from build123d import *

# Parameters (mm, degrees)
SKETCH1_R           = 1.4986
BOSS_EXTRUDE1_DEPTH = 6.731
BOSS_EXTRUDE2_DEPTH = 2.54
SKETCH3_W           = 2.54
SKETCH3_H           = 3.283466221
BOSS_EXTRUDE3_DEPTH = 8.0264


with BuildPart() as part:
    # Sketch1 → Boss-Extrude1 (new body)
    with BuildSketch(Plane.XY):
        Circle(SKETCH1_R)
    extrude(amount=BOSS_EXTRUDE1_DEPTH)

    # Sketch2 → Boss-Extrude2 (add)
    with BuildSketch(Plane(origin=(0, 0, 0), x_dir=(-1, 0, 0), z_dir=(0, 0, -1))):
        with BuildLine():
            Line((-1.74748007, -0.387866221), (-2.463536443, -0.387866221))
            ThreePointArc((-2.463536443, -0.387866221), (-2.643141566, -0.313471343), (-2.717536443, -0.133866221))
            Line((-2.717536443, -0.133866221), (-2.717536443, 3.1496))
            ThreePointArc((-2.717536443, 3.1496), (-2.345562055, 4.047625612), (-1.447536443, 4.4196))
            Line((-1.447536443, 4.4196), (1.417916008, 4.4196))
            ThreePointArc((1.417916008, 4.4196), (2.312179766, 4.051371774), (2.687871622, 3.160217845))
            Line((2.687871622, 3.160217845), (2.715395045, -0.131742652))
            ThreePointArc((2.715395045, -0.131742652), (2.641758277, -0.312718973), (2.461403923, -0.387866221))
            Line((2.461403923, -0.387866221), (1.74748007, -0.387866221))
            ThreePointArc((1.74748007, -0.387866221), (1.561141898, -0.306475854), (1.494222089, -0.114465319))
            ThreePointArc((1.494222089, -0.114465319), (0, 1.4986), (-1.494222089, -0.114465319))
            ThreePointArc((-1.494222089, -0.114465319), (-1.561141898, -0.306475854), (-1.74748007, -0.387866221))
        make_face()
    extrude(amount=-BOSS_EXTRUDE2_DEPTH)

    # Sketch3 → Boss-Extrude3 (add)
    with BuildSketch(Plane(origin=(2.717536443, 0, 0), x_dir=(0, 0, -1), z_dir=(1, 0, 0))):
        with Locations((-1.27, 1.50786689)):
            Rectangle(SKETCH3_W, SKETCH3_H)
    extrude(amount=BOSS_EXTRUDE3_DEPTH)

    # Mirror4: part across plane


with BuildPart() as part_1:
    add(part.part)
    add(part.part.mirror(Plane(origin=(10.743936443, 0, 0), x_dir=(0, 0, 1), z_dir=(1, 0, 0))))


solid = part_1.part
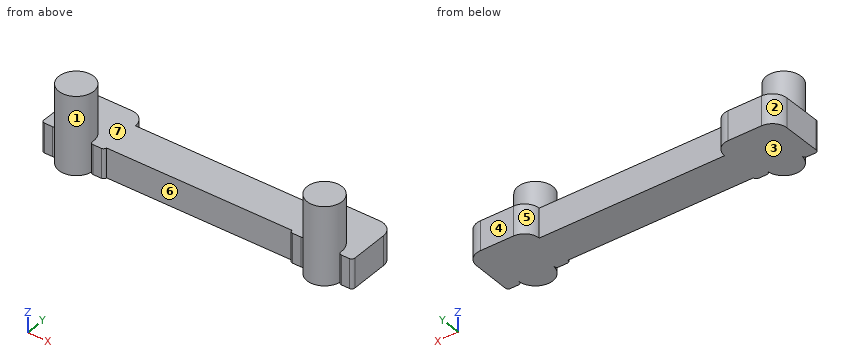
Input: part model. Units: mm. Frame: model coordinates. Face numbers are marked on the shaded views. A direction names the side the tool comes from. Coordinates: 2 decimals unless noted, no trailing zeros. Loops run counter-clockwise (first coordinate to the right, second up) from the corner with the lowest first, then second, coordinate; pieces in that order, holes last. Notation, with made-up numbers: (-14.5, -29.75) -> (1.5, -29.75) arc R27 cw to (1.5, 3.25) -> close; hole circle Ø5 at (-16.75, -33.75). An arc over 180 degrees is marked (long way). Write each question's results on one line, items separated by ' | '. Start each with the question number.
Q1. Pin query (flat end, axial travel): pin 1 (1.4 mm diameter, centred on x = 4, y = 3, fed in from +Z); pin 2 (2 mm diameter, centred on x = 8.5, z = 1.5, fed in from +Y); pin 3 (2 mm diameter, centred on x = 9.5, z = 1, fed in from -Y). Return the tip coordinate at first contact, or that it passes through.
Q2. Section B-B, the plane z = 4.5. Return the cut outline in (x, y), plus the area to 3 significant figures.
Q3. Section A-A, the plane y = 3.55. Return the cut outline in (x, z), plus the area to 3 significant figures.
Q4. Ray query, line 1 (X direction, y = 3.25, z = 0.5); line 2 (Y direction, x = 14, z = 2); line 3 (X direction, y = 1.3, z = 4.5). Return the intervals inside material, ascending. Write a range as from..to.
Q5. Section D-D, the plane z = 2.25. Return the cut outline in (x, y), plus the area to 3 significant figures.
Q6. Pull-direction query (X, two-part tool) for the marked faces 1, 2 and 3; classes: released by +X, released by -X, zero draft, split by the parting line, or undercut.
Q7. Section C-C, the plane x = 17.5. Return the cut outline in (y, z), plus the area to 3 significant figures.
Q8. Reachability of the marked faces 4, 5, 6 and 7 from +Z, -Z, +X, -X, +Y, -Y: full face, straight path, thin tool, end or side. Return the list, or none.
Found:
1) pin 1: z = 2.54 | pin 2: y = 3.15 | pin 3: y = -0.13
2) outline: circle Ø3 at (0, 0); circle Ø3 at (21.49, 0) | area: 14.1 mm2
3) outline: (-2.62, 0) -> (2.65, 0) -> (2.65, 2.54) -> (-2.62, 2.54) -> close; (18.84, 0) -> (24.11, 0) -> (24.11, 2.54) -> (18.84, 2.54) -> close | area: 26.8 mm2
4) line 1: -2.68..2.71, 18.77..24.17 | line 2: -0.13..3.15 | line 3: -0.75..0.75, 20.74..22.23
5) outline: (-2.72, -0.13) arc R0.25 ccw to (-2.46, -0.39) -> (-1.75, -0.39) arc R0.25 ccw to (-1.49, -0.11) arc R1.5 ccw to (1.49, -0.11) arc R0.25 ccw to (1.75, -0.39) -> (2.46, -0.39) arc R0.25 ccw to (2.72, -0.13) -> (18.77, -0.13) arc R0.25 ccw to (19.02, -0.39) -> (19.74, -0.39) arc R0.25 ccw to (19.99, -0.11) arc R1.5 ccw to (22.98, -0.11) arc R0.25 ccw to (23.24, -0.39) -> (23.95, -0.39) arc R0.25 ccw to (24.2, -0.13) -> (24.18, 3.16) arc R1.27 ccw to (22.91, 4.42) -> (20.04, 4.42) arc R1.27 ccw to (18.77, 3.15) -> (2.72, 3.15) arc R1.27 ccw to (1.45, 4.42) -> (-1.42, 4.42) arc R1.27 ccw to (-2.69, 3.16) -> close | area: 108 mm2
6) face 1: undercut | face 2: released by -X | face 3: zero draft
7) outline: (-0.13, 0) -> (3.15, 0) -> (3.15, 2.54) -> (-0.13, 2.54) -> close | area: 8.34 mm2
8) face 4: +Z, -Z, +X, -X, +Y | face 5: +Z, -Z, +Y | face 6: +Z, -Z, -Y | face 7: +Z, +Y
